```python
from build123d import *

# Parameters (mm, degrees)
ESBO_O1_R                                   = 9.1
RESSALTO_EXTRUS_O1_DEPTH                    = 3
ESBO_O2_R                                   = 6.7
RESSALTO_EXTRUS_O2_DEPTH                    = 87
FURO_ROSCADO_PARA_CONDU_TE_DE_M4X0_72_D     = 4.2
FURO_ROSCADO_PARA_CONDU_TE_DE_M4X0_72_DEPTH = 22
FURO_ROSCADO_PARA_CONDU_TE_DE_M4X0_72_TIP   = 1.2618073


with BuildPart() as part:
    # Esboço1 → Ressalto-extrusão1 (new body)
    with BuildSketch(Plane.XY):
        Circle(ESBO_O1_R)
    extrude(amount=-RESSALTO_EXTRUS_O1_DEPTH)

    # Esboço2 → Ressalto-extrusão2 (add)
    with BuildSketch(Plane(origin=(0, 0, -3), x_dir=(-1, 0, 0), z_dir=(0, 0, -1))):
        Circle(ESBO_O2_R)
    extrude(amount=RESSALTO_EXTRUS_O2_DEPTH)

    # Furo roscado para conduíte de M4x0.72
    with Locations(Plane(origin=(0, 0, -90), x_dir=(-1, 0, 0), z_dir=(0, 0, -1))):
        with Locations((0, 0)):
            Hole(FURO_ROSCADO_PARA_CONDU_TE_DE_M4X0_72_D / 2, depth=FURO_ROSCADO_PARA_CONDU_TE_DE_M4X0_72_DEPTH)
            with Locations((0, 0, -(FURO_ROSCADO_PARA_CONDU_TE_DE_M4X0_72_DEPTH + FURO_ROSCADO_PARA_CONDU_TE_DE_M4X0_72_TIP / 2))):  # 118° drill point
                Cone(0, FURO_ROSCADO_PARA_CONDU_TE_DE_M4X0_72_D / 2, FURO_ROSCADO_PARA_CONDU_TE_DE_M4X0_72_TIP, mode=Mode.SUBTRACT)


solid = part.part
```
Source: CAD feature listing. Evaluate the final solid. Frame: model axes, mm. A direction names the side the tool comes from. Give positions to 0.01 mm unless a question says otherwise; leave off trailing zeros. Order: outer loops, then holes, each group sorted by start corner. A loop starts at its lowest first (then second) coordinate and runs counter-clockwise, first axis right, second up. Notation, with made-up numbers: (66, 50) -> (102, 50) arc R32 ccw to (102, 87) -> close; hole circle Ø4 at (18.25, 89). An arc over 180 degrees is marked (long way). Use a Markdown table: item, result.
Q1. Section A-A (x = 4.75). Return the cut outline in (y, z).
A:
| item | result |
|---|---|
| outline | (-7.76, -3) -> (-4.73, -3) -> (-4.73, -90) -> (4.73, -90) -> (4.73, -3) -> (7.76, -3) -> (7.76, 0) -> (-7.76, 0) -> close |
Q2. Material intervals for line 1 (Y direction, x = 0, z = -72.5); line 2 (Z direction, x = 1.75, y = 7); line 3 (X direction, y = 0.5, z = -9), sorted ascending. Write a range as [from, to].
A:
| item | result |
|---|---|
| line 1 | [-6.7, -2.1], [2.1, 6.7] |
| line 2 | [-3, 0] |
| line 3 | [-6.68, 6.68] |
Q3. Access query for faces 4 (the face through (2, 2, -90)), 5 (the face through (2.003, 0.631, -78.846)). Directions: +Z, -Z, +X, -X, +Y, -Y. A direction counts if a zero-diameter tool reaches every point of the face in a straight line with its end or side. Return the directions, or none.
A:
| item | result |
|---|---|
| face 4 | -Z, +X, -X, +Y, -Y |
| face 5 | -Z |
Q4. Pull-direction query (Y, two-part tool) for faces 1 (the face through (0, 0, 0)), 2 (the face through (-0.35, 0.11, -66.96)), 3 (the face through (-1.973, -8.884, -1.479)); classes: +Y half, -Y half, draft (parallel to the pull), parting line (faces both ways), or undercut.
A:
| item | result |
|---|---|
| face 1 | draft |
| face 2 | undercut |
| face 3 | parting line |
Q5. Section C-C (z = -80). Return the cut outline in (x, y), and give its area (3 significant figures).
A:
| item | result |
|---|---|
| outline | circle Ø13.4 at (0, 0); hole circle Ø4.2 at (0, 0) |
| area | 127 mm^2 |
Q6. Section B-B (y = 3.25). Return the cut outline in (x, z), and give its area (3 significant figures).
A:
| item | result |
|---|---|
| outline | (-8.5, -3) -> (-5.86, -3) -> (-5.86, -90) -> (5.86, -90) -> (5.86, -3) -> (8.5, -3) -> (8.5, 0) -> (-8.5, 0) -> close |
| area | 1,070 mm^2 |
Q7. Section D-D (z = -59.5). Return the cut outline in (x, y).
A:
| item | result |
|---|---|
| outline | circle Ø13.4 at (0, 0) |
Q8. First-contact query: P1, Ø1.5, axis at x = -2.5, z = -15, coming from the -Y side; P2, Ø2, axis at x = -5.5, z = -9, coming from the +Y side; P3, Ø3, axis at y = 3, z = -38, coming from the +X side. Flat tips, straight axial feed; report the tip coordinate or a pass-through.
A:
| item | result |
|---|---|
| P1 | y = -6.47 |
| P2 | y = 4.96 |
| P3 | x = 6.53 |
